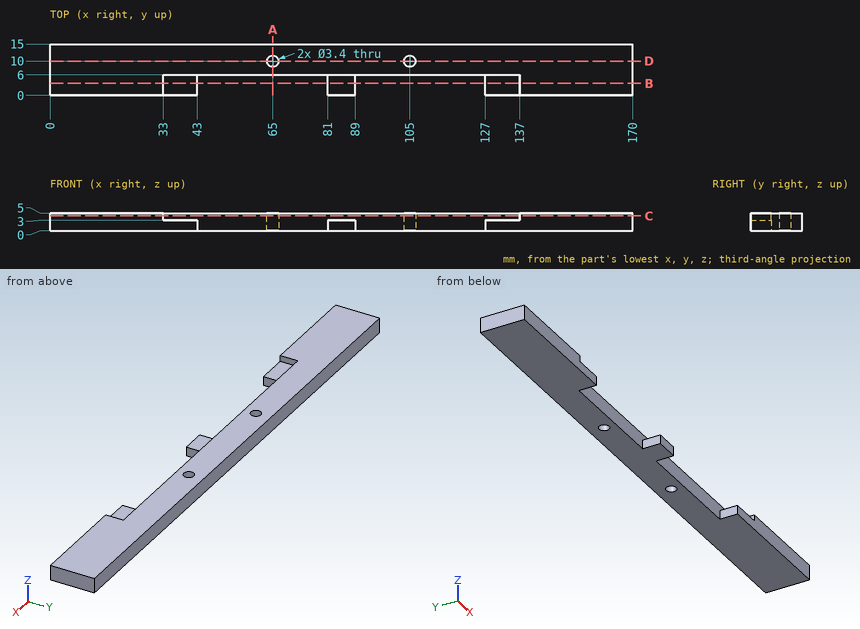
Can you work these out from the drawing? Everything is in mm from the part's minimum corner. Round coordinates to 2 decimals unless told otherwise and drop trailing zeros. Write each loop counter-clockwise with the first axis right and the second up, starting at its lowest first coordinate (ties: lowest second). Pieces come first, ordered by that corner, then holes. Notation, with made-up numbers: M -0.75,67.25 L 57.25,67.25 A26 ccw 57.25,97.25 Z; hole C 65.25,-13 d2. An arc over 180 degrees is marked long. Use a Markdown table: item, result.
Item 1: If I drill on line 1 along X through (y, z) = (4, 2.3); line 2 along Y through (x, z) = (65, 3.45); line 3 along X through (y, z) = (4.75, 4.5), over which ranges is the centre line in solid material (lowest first)? Write a range as [from, to].
Found:
| item | result |
|---|---|
| line 1 | x = [0, 43], [81, 89], [127, 170] |
| line 2 | y = [6, 8.3], [11.7, 15] |
| line 3 | x = [0, 33], [137, 170] |
Item 2: I want a section at A-A (x = 65). List the corners of the cut face in (y, z) for me, and give its area (3 significant figures).
Found:
| item | result |
|---|---|
| outline | M 6,0 L 8.3,0 L 8.3,5 L 6,5 Z; M 11.7,0 L 15,0 L 15,5 L 11.7,5 Z |
| area | 28.0 mm2 |
Item 3: For pin 1 Ø1 at (x, z) = (109, 1.5) entering from -Y; pin 2 Ø1.5 at (y, z) = (4.5, 1) entering from -X; pin 3 Ø1.8 at (x, y) = (39, 1.5) entering from +Z; pin 4 Ø3 at (x, y) = (105, 10) entering from +Z, each with a flat end and sliding along its axis, tell me the tip position at first contact or that it passes through.
Found:
| item | result |
|---|---|
| pin 1 | stops at y = 6 |
| pin 2 | stops at x = 0 |
| pin 3 | stops at z = 3 |
| pin 4 | passes through |
Item 4: I want a section at B-B (y = 3.5). List the corners of the cut face in (x, z) for me, and give its area (3 significant figures).
Found:
| item | result |
|---|---|
| outline | M 0,0 L 43,0 L 43,3 L 33,3 L 33,5 L 0,5 Z; M 81,0 L 89,0 L 89,3 L 81,3 Z; M 127,0 L 170,0 L 170,5 L 137,5 L 137,3 L 127,3 Z |
| area | 414 mm2 |
Item 5: I want a section at D-D (y = 10). List the corners of the cut face in (x, z) for me, and give its area (3 significant figures).
Found:
| item | result |
|---|---|
| outline | M 0,0 L 63.3,0 L 63.3,5 L 0,5 Z; M 66.7,0 L 103.3,0 L 103.3,5 L 66.7,5 Z; M 106.7,0 L 170,0 L 170,5 L 106.7,5 Z |
| area | 816 mm2 |
Item 6: I want a section at C-C (z = 4.25). List the corners of the cut face in (x, y) for me, and give its area (3 significant figures).
Found:
| item | result |
|---|---|
| outline | M 0,0 L 33,0 L 33,6 L 137,6 L 137,0 L 170,0 L 170,15 L 0,15 Z; hole C 65,10 d3.4; hole C 105,10 d3.4 |
| area | 1,910 mm2 |
